CAD build for the part. Positions are in the model's coordinates, mm. A direction names the side the tool comes from. Coordinates: 2 decimals unless noted, no trailing zeros. Order: outer loops, then holes, each group sorted by start corner. A loop starts at its lowest first (then second) coordinate and runs counter-clockwise, first axis right, second up. Notation, with made-up numbers: (53.25, 58) - (102.25, 58) arc R14 ccw to (102.25, 75) - close; hole circle Ø4 at (-38.5, 84). An arc over 180 degrees is marked (long way). Return JSON: item names as keys, results as strings.
from build123d import *

# Parameters (mm, degrees)
SKETCH_1_R      = 1.3
EXTRUDE_1_DEPTH = 3


with BuildPart() as part:
    # 草图1 → 凸台-拉伸1 (new body)
    with BuildSketch(Plane(origin=(0, 0, -3.362857667), x_dir=(-1, 0, 0), z_dir=(0, 0, -1))):
        with BuildLine():
            Line((-6.304159928, 7.933833034), (-4.539684391, 14.518557193))
            ThreePointArc((-4.539684391, 14.518557193), (-3.62301138, 15.532716808), (-2.264294404, 15.382060533))
            Line((-2.264294404, 15.382060533), (-0.142530428, 17.503217342))
            Line((-0.142530428, 17.503217342), (4.099819599, 13.25965297))
            Line((4.099819599, 13.25965297), (5.796991646, 14.956339352))
            Line((5.796991646, 14.956339352), (1.554014804, 19.200530718))
            Line((1.554014804, 19.200530718), (3.675778781, 21.321687528))
            Line((3.675778781, 21.321687528), (-4.808443123, 29.808337985))
            Line((-4.808443123, 29.808337985), (-6.931968366, 27.685420414))
            Line((-6.931968366, 27.685420414), (-11.174318393, 31.928984786))
            Line((-11.174318393, 31.928984786), (-12.870428791, 30.231215419))
            Line((-12.870428791, 30.231215419), (-8.629080401, 25.98865297))
            Line((-8.629080401, 25.98865297), (-10.750844377, 23.867496161))
            Line((-10.750844377, 23.867496161), (-10.611098311, 23.731253658))
            ThreePointArc((-10.611098311, 23.731253658), (-8.929299443, 20.817545637), (-8.929456987, 17.45330102))
            Line((-8.929456987, 17.45330102), (-12.208534908, 5.216337034))
            ThreePointArc((-12.208534908, 5.216337034), (-8.203956956, -0.691485495), (-5.819308033, 6.03550946))
            ThreePointArc((-5.819308033, 6.03550946), (-6.310108859, 6.921233679), (-6.304159928, 7.933833034))
        make_face()
        with Locations(Location((-8.71249984, 3.274951558, 0), (0, 0, 180))):
            Circle(SKETCH_1_R, mode=Mode.SUBTRACT)
        with Locations(Location((-3.536567574, 22.593983824, 0), (0, 0, 180))):
            Circle(SKETCH_1_R, mode=Mode.SUBTRACT)
    extrude(amount=-EXTRUDE_1_DEPTH)


solid = part.part
Item 1: Mould opens along X. For faces 1 (the flat face through (9.68, 24.94, -1.88)), 2 (the flat face through (1, 26, -2)), 3 (the cylindrical face through (3.642, 15.526, -1.884)) say: released by +X, released by -X, zero draft, split by the parting line, or undercut.
Findings below:
{"face 1": "released by +X", "face 2": "released by -X", "face 3": "undercut"}
Item 2: Band-saw the part on B-B, the plane x = -2. List the corners of the cut face in (y, z), then the cut area to 3 significant figures.
Findings below:
{"outline": "(15.36, -3.36) - (18.75, -3.36) - (18.75, -0.36) - (15.36, -0.36) - close; (19.65, -3.36) - (23, -3.36) - (23, -0.36) - (19.65, -0.36) - close", "area": "20.2 mm²"}
Item 3: Band-saw the part on C-C, the plane z = -2.2. List the corners of the cut face in (x, y), then the cut area to 3 significant figures.
Findings below:
{"outline": "(-5.8, 14.96) - (-4.1, 13.26) - (0.14, 17.5) - (2.26, 15.38) arc R1.5 cw to (4.54, 14.52) - (6.3, 7.93) arc R2 cw to (5.82, 6.04) arc R4 ccw (long way) to (12.21, 5.22) - (8.93, 17.45) arc R6.5 cw to (10.61, 23.73) - (10.75, 23.87) - (8.63, 25.99) - (12.87, 30.23) - (11.17, 31.93) - (6.93, 27.69) - (4.81, 29.81) - (-3.68, 21.32) - (-1.55, 19.2) - close; hole circle Ø2.6 at (3.54, 22.59); hole circle Ø2.6 at (8.71, 3.27)", "area": "236 mm²"}
Item 4: Band-saw the part on D-D, the plane y = 20. List the corners of the cut face in (x, z), then the cut area to 3 significant figures.
Findings below:
{"outline": "(-2.35, -3.36) - (8.77, -3.36) - (8.77, -0.36) - (-2.35, -0.36) - close", "area": "33.4 mm²"}
Item 5: Band-saw the part on A-A, the plane y = 28. List the corners of the cut face in (x, z).
Findings below:
{"outline": "(3, -3.36) - (6.62, -3.36) - (6.62, -0.36) - (3, -0.36) - close; (7.25, -3.36) - (10.64, -3.36) - (10.64, -0.36) - (7.25, -0.36) - close"}
Item 6: Drop flat-ended pins along their axis: P1, Ø3.5, axis at x = 3.54, y = 22.59, coming from the -Z side; P2, Ø1.5, axis at x = 10, z = -3, coming from the -Y side. Give the stop position or say it passes through.
Findings below:
{"P1": "stops at z = -3.36", "P2": "stops at y = -0.69"}
Item 7: Wall check: L1, parallel to Y at x = 8.5, z = -0.6; L2, parallel to X at y = 28.5, z = -2.4; L3, parallel to Y at x = 3, z = -2.35. Give the ranges that are in metal, low to high. Write a range as [from, to].
Findings below:
{"L1": "y = [-0.72, 1.99], [4.56, 29.25]", "L2": "x = [3.5, 6.12], [7.75, 11.14]", "L3": "y = [15.63, 21.41], [23.78, 28]"}
Item 8: Which spindle directions (+Z, -Z, +X, -X, +Y, -Y) get a long thin tool onto all of the face, cutting with end or side? Do faces 4 (the flat face through (5.434, 11.18, -1.884)), 5 (the flat face through (-1.95, 15.41, -1.88)), 6 (the flat face through (10.78, 28.14, -1.88)), 7 (the flat face through (5.855, 28.762, -1.884)), 8 (the flat face through (-2.6, 20.246, -1.884)). Say none if no direction does.
Findings below:
{"face 4": "+Z, -Z", "face 5": "+Z, -Z, -Y", "face 6": "+Z, -Z, +X", "face 7": "+Z, -Z, +Y", "face 8": "+Z, -Z, -X"}
